Model file for the job. Use its own axes, mm. Coordinates: 2 decimals unless noted, no trailing zeros. Loops run counter-clockwise (first coordinate to the right, second up) from the corner with the lowest first, then second, coordinate; pieces in that order, holes last.
Autodesk Inventor part; units mm, degrees
ref_plane "YZ Plane" through (0, 0, 0) normal (1, 0, 0) x (0, 1, 0)
ref_plane "XZ Plane" through (0, 0, 0) normal (0, 1, 0) x (-1, 0, 0)
ref_plane "XY Plane" through (0, 0, 0) normal (0, 0, 1) x (1, 0, 0)
sketch "Szkic1" plane through (0, 0, 0) normal (0, 1, 0) x (-1, 0, 0)
  circle A0 centre (0, 0) radius 30
  dimension "d0" = 60
extrude "Wyciągnięcie proste1" add sketch "Szkic1" along normal blind 15
sketch "Szkic2" plane through (0, 15, 0) normal (0, 1, 0) x (1, 0, 0)
  circle A0 centre (0, 0) radius 30
  circle A1 centre (0, 0) radius 1.5
  dimension "d3" = 3
hole "Otwór1" at (0, 15, 0) direction (0, -1, 0) diameter 3 depth 15 tip angle 118
chamfer "Faza1" distance 0.2 angle 45 1 edges at (0, 15, -1.5)
chamfer "Faza2" distance 0.2 angle 45 1 edges at (0, 0, -1.5)
properties part number "koło" material "Żywica acetalowa, czarna"
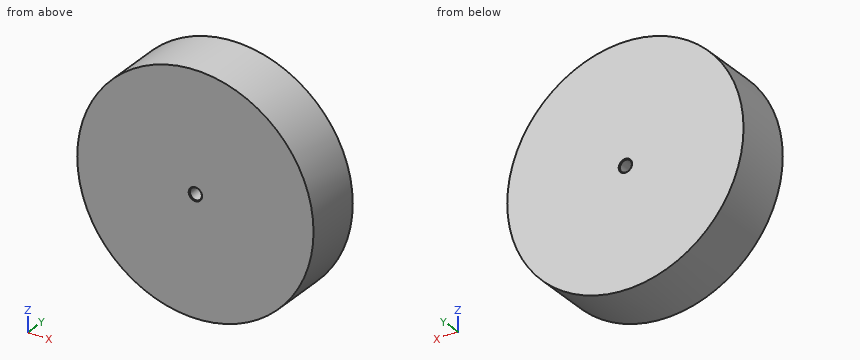
Q1. Flat gauge pins, fed straight in: P1, Ø8, axis at x = 3, y = 8, coming from the +Z side; P2, Ø1, axis at x = -17.5, y = 13, coming from the +Z side; P3, Ø5, axis at y = 6.5, z = 7, coming from the +X side. Where does each tip first touch, or does it go through?
Answers:
P1: stops at z = 30
P2: stops at z = 24.72
P3: stops at x = 29.66
Q2. Slice it at B-B (z = 0). List the corners of the cut face in (x, y).
Answers:
outline: (-30, 0) - (-1.7, 0) - (-1.5, 0.2) - (-1.5, 14.8) - (-1.7, 15) - (-30, 15) - close; (1.5, 0.2) - (1.7, 0) - (30, 0) - (30, 15) - (1.7, 15) - (1.5, 14.8) - close
Q3. Slice it at C-C (y = 9.75). List the corners of the cut face in (x, z).
Answers:
outline: circle Ø60 at (0, 0); hole circle Ø3 at (0, 0)
Q4. Drill centre lines: line 1 (Z direction, x = 0, y = 10); line 2 (Z direction, x = -2.5, y = 2); line 3 (X direction, y = 14.25, z = -7). Where is each one in solid material? Low to high.
Answers:
line 1: z = -30 to -1.5, 1.5 to 30
line 2: z = -29.9 to 29.9
line 3: x = -29.17 to 29.17
Q5. Slice it at A-A (x = 0). List the corners of the cut face in (y, z), and give its area (3 significant figures).
Answers:
outline: (0, -30) - (15, -30) - (15, -1.7) - (14.8, -1.5) - (0.2, -1.5) - (0, -1.7) - close; (0, 1.7) - (0.2, 1.5) - (14.8, 1.5) - (15, 1.7) - (15, 30) - (0, 30) - close
area: 855 mm2
Q6. Slice it at D-D (z = 21.5). List the corners of the cut face in (x, y).
Answers:
outline: (-20.92, 0) - (20.92, 0) - (20.92, 15) - (-20.92, 15) - close
